Autodesk Inventor part; units mm, degrees
ref_plane "YZ Plane" through (0, 0, 0) normal (1, 0, 0) x (0, 1, 0)
ref_plane "XZ Plane" through (0, 0, 0) normal (0, 1, 0) x (-1, 0, 0)
ref_plane "XY Plane" through (0, 0, 0) normal (0, 0, 1) x (1, 0, 0)
sketch "Sketch1" plane through (0, 0, 0) normal (0, 1, 0) x (-1, 0, 0)
  line L0 (0, 0) -> (24, 0)
  line L1 (24, 0) -> (24, 64)
  line L2 (24, 64) -> (0, 64)
  line L3 (0, 64) -> (0, 0)
  dimension "d0" = 24
  dimension "d1" = 64
extrude "Extrusion1" add sketch "Sketch1" along normal blind 1
sketch "Sketch2" plane through (0, 0, 0) normal (0, -1, 0) x (1, 0, 0)
  line L0 (-24, 0) -> (-24, 64)
  line L1 (0, 0) -> (-24, 0)
  line L2 (0, 64) -> (0, 0)
  line L3 (-24, 64) -> (0, 64)
  line L4 (-2, 2) -> (-22, 2)
  line L5 (-22, 2) -> (-22, 62)
  line L6 (-22, 62) -> (-2, 62)
  line L7 (-2, 62) -> (-2, 2)
  line L8 (-4, 4) -> (-20, 4)
  line L9 (-20, 4) -> (-20, 60)
  line L10 (-20, 60) -> (-4, 60)
  line L11 (-4, 60) -> (-4, 4)
  dimension "d4" = 2
  dimension "d5" = 2
extrude "Extrusion2" add sketch "Sketch2" along normal blind 5 contours L4 L5 L6 L7
sketch "Sketch3" plane through (0, 0, 0) normal (0, -1, 0) x (1, 0, 0)
  line L0 (-4, 4) -> (-4, 60)
  line L1 (-4, 60) -> (-20, 60)
  line L2 (-20, 60) -> (-20, 4)
  line L3 (-20, 4) -> (-4, 4)
  line L4 (-4, 4) -> (-20, 4) construction
  line L5 (-12, 4) -> (-12, 60) construction
  line L6 (-4, 60) -> (-20, 60) construction
  line L7 (-12, 4) -> (-12, 5) construction
  line L8 (-12, 60) -> (-12, 59) construction
  line L9 (-12, 59) -> (-12, 50) construction
  line L10 (-12, 50) -> (-12, 41) construction
  line L11 (-12, 41) -> (-12, 32) construction
  line L12 (-12, 32) -> (-12, 23) construction
  line L13 (-12, 23) -> (-12, 14) construction
  circle A0 centre (-12, 50) radius 2.5
  circle A1 centre (-12, 41) radius 2.5
  circle A2 centre (-12, 32) radius 2.5
  circle A3 centre (-12, 23) radius 2.5
  circle A4 centre (-12, 14) radius 2.5
  point P0 (0, 0)
  dimension "d8" = 1
  dimension "d9" = 1
  dimension "d10" = 9
  dimension "d11" = 9
  dimension "d12" = 9
  dimension "d13" = 9
  dimension "d14" = 9
  dimension "d15" = 5
  dimension "d16" = 5
  dimension "d17" = 5
  dimension "d18" = 5
  dimension "d19" = 5
extrude "Extrusion3" cut sketch "Sketch3" against normal blind 2 contours A0 | A1 | A2 | A3 | A4
properties part number "Parte 2.2 final"
Design review of the part built by this model. Coordinates are the model's own, in mm. A direction names the side the tool comes from. Round coordinates to 2 decimals unless told otherwise and drop trailing zeros. Order: outer loops, then holes, each group sorted by start corner. A loop starts at its lowest first (then second) coordinate and runs counter-clockwise, first axis right, second up. Notation, with made-up numbers: (-10.75, 12) - (-6.75, 12) arc R22 cw to (-6.75, 26) - close; hole circle Ø9 at (-36.75, 8.25). An arc over 180 degrees is marked (long way). Return JSON: item names as keys, results as strings.
Q1. Consider section C-C on y = -1.95. Write out the cut boundary in (x, z), plus the area to 3 significant figures.
Computed values:
{"outline": "(-22, 2) - (-2, 2) - (-2, 62) - (-22, 62) - close; hole (-20, 4) - (-4, 4) - (-4, 60) - (-20, 60) - close", "area": "304 mm2"}
Q2. Consider section A-A on z = 32. Write out the cut boundary in (x, y), plus the area to 3 significant figures.
Computed values:
{"outline": "(-24, 0) - (-22, 0) - (-22, -5) - (-20, -5) - (-20, 0) - (-14.5, 0) - (-14.5, 1) - (-24, 1) - close; (-9.5, 0) - (-4, 0) - (-4, -5) - (-2, -5) - (-2, 0) - (0, 0) - (0, 1) - (-9.5, 1) - close", "area": "39.0 mm2"}
Q3. The part is to be moulded in two halves that separate along Z. For faces 1 (the cylindrical face through (-12.54, 0.49, 38.56)), 2 (the flat face through (-12, -2, 2)), 3 (the flat face through (-1, 0, 35)), 4 (the flat face through (-12, -2, 62)), say which applies: pulls with the +Z half, pulls with the -Z half, needs draft (parallel to the pull), parting line crosses it, or undercut.
Computed values:
{"face 1": "undercut", "face 2": "pulls with the -Z half", "face 3": "needs draft", "face 4": "pulls with the +Z half"}
Q4. Consider section B-B on x = -12. Give the number of separate pieces and of enclosed holes in the cut face, plus the area to 3 significant figures.
Computed values:
{"separate pieces": "6", "enclosed holes": "0", "area": "59.0 mm2"}
Q5. Consider section D-D on x = -18.75. Write out the cut boundary in (y, z), plus the area to 3 significant figures.
Computed values:
{"outline": "(-5, 2) - (0, 2) - (0, 0) - (1, 0) - (1, 64) - (0, 64) - (0, 62) - (-5, 62) - (-5, 60) - (0, 60) - (0, 4) - (-5, 4) - close", "area": "84.0 mm2"}
Q6. Wall thickness on L1, parallel to Z at x = -12, y = 0.5; L2, parallel to X at y = -4.1, z = 22.5; L3, parallel to Z at x = -18.5, y = -0.95: over which ranges is each line inside the solid? List them lowest first. Write a range as [from, to].
Computed values:
{"L1": "z = [0, 11.5], [16.5, 20.5], [25.5, 29.5], [34.5, 38.5], [43.5, 47.5], [52.5, 64]", "L2": "x = [-22, -20], [-4, -2]", "L3": "z = [2, 4], [60, 62]"}
Q7. Machinability: for faces 5 (the flat face through (-22, -2, 32)), 6 (the flat face through (-2, -2, 32)), 7 (the flat face through (-12, -2, 4)), which of the approach directions +Z, -Z, +X, -X, +Y, -Y give a long, thin tool a straight path to every point of the face, cutting with its end or side? Answer none if there is none.
Computed values:
{"face 5": "+Z, -Z, -X, -Y", "face 6": "+Z, -Z, +X, -Y", "face 7": "-Y"}
Q8. For pin 1 Ø4 at (x, z) = (-12, 14) entering from -Y; pin 2 Ø5 at (x, z) = (-16, 27.5) entering from -Y; pin 3 Ø2.5 at (x, y) = (-13.5, -2.5) entering from -Z; pin 4 Ø3 at (y, z) = (-3, 46.5) entering from -X, all flat-tipped, find the tip position at first contact; note any pin that passes through.
Computed values:
{"pin 1": "passes through", "pin 2": "stops at y = 0", "pin 3": "stops at z = 2", "pin 4": "stops at x = -22"}
